Can you work these out from the model? Positions are in its coordinate system, mm. A direction names the side the tool comes from. Round coordinates to 2 decimals unless told otherwise and drop trailing zeros. Loops run counter-clockwise (first coordinate to the right, second up) from the corner with the lowest first, then second, coordinate; pieces in that order, holes last.
(1) Thinking about a two-plate mould opening in Y: for faces 5 (the face through (-2, 50.8, 135)), 6 (the face through (-2, 49, 19.05)), 7 (the face through (1.6, 47.6, 69)), which applies, released by +Y, released by -Y, zero draft, split by the parting line, or undercut?
(2) If I drill on line 1 along Z through (x, y) = (25, 34) (3 decimals); line 2 along Z through (x, y) = (38.5, 17) (3 decimals); line 3 along X through (y, z) = (3, 25) (3 decimals), over which ranges is the centre line in solid material (lowest first)?
(3) I want a section at A-A on z = 100. Write out the boundary of the cut face in (x, y) (3 decimals).
(4) Will these pins go through, and if not, where does the flat tip stop? pin 1 Ø1.9 at (x, z) = (25, 135.5) entering from +Y; pin 2 Ø4 at (x, z) = (26.5, 124) entering from +Y (3 decimals); pin 3 Ø1.6 at (y, z) = (49.5, 12.5) entering from -X.
(5) Which directions (+Z, -Z, +X, -X, +Y, -Y) give clear straight access to the entire face, cutting with the end or side of a thin tool? Please do faces 1 (the face through (-6, 25, 134.938)), 2 (the face through (22, 20.671, 135)), 3 (the face through (-2, 47.625, 97)), 4 (the face through (-6, 44.45, 137)).
(6) I want a section at C-C on x = 25.4. Write out the boundary of the cut face in (y, z) (1 decimal).
(7) I want a section at D-D on x = 42. Write out the boundary of the cut face in (y, z) (3 decimals), plus the area to 3 significant figures.
(8) I want a section at B-B on y = 28. Write out the boundary of the cut face in (x, z) (1 decimal).
from build123d import *

# Parameters (mm, degrees)
BOSS_EXTRUDE1_DEPTH = 139.7
SHELL1_T            = -3.175
BOSS_EXTRUDE2_START = -9.525
BOSS_EXTRUDE2_DEPTH = 9.525
BOSS_EXTRUDE3_DEPTH = 9.525
SKETCH5_W           = 139.7
SKETCH5_H           = 50.8
SKETCH5_W_2         = 120.65
SKETCH5_H_2         = 44.45
BOSS_EXTRUDE4_DEPTH = 3.175
SKETCH6_W           = 3.175
SKETCH6_H           = 38.1
BOSS_EXTRUDE5_DEPTH = 5.08
CUT_EXTRUDE1_REACH  = 159.09
SKETCH7_W           = 3.175
SKETCH7_H           = 9.525
SKETCH9_W           = 47.625
SKETCH9_H           = 120.65
CUT_EXTRUDE2_DEPTH  = 157.092506627
SKETCH8_R           = 0.75
BOSS_EXTRUDE6_DEPTH = 9
SKETCH10_W          = 25.4
SKETCH10_H          = 9.525
CUT_EXTRUDE3_DEPTH  = 149.683592319
SKETCH11_R          = 1.905
CUT_EXTRUDE4_DEPTH  = 25.4


with BuildPart() as part:
    # Sketch1 → Boss-Extrude1 (new body)
    with BuildSketch(Plane.XY):
        with BuildLine():
            Line((0, 0), (0, 50.8))
            ThreePointArc((0, 50.8), (35.921024484, 35.921024484), (50.8, 0))
            Line((50.8, 0), (0, 0))
        make_face()
    extrude(amount=BOSS_EXTRUDE1_DEPTH)

    # Shell1
    shell1_openings = [part.faces().sort_by_distance(p)[0] for p in [
        (0, 25.4, 69.85),
    ]]
    offset(amount=SHELL1_T, openings=shell1_openings, kind=Kind.INTERSECTION)

    # Sketch3 → Boss-Extrude2 (add)
    with BuildSketch(Plane.XY.offset(139.7).offset(BOSS_EXTRUDE2_START)):
        with BuildLine():
            Line((0, 50.8), (0, 0))
            Line((0, 0), (50.8, 0))
            ThreePointArc((50.8, 0), (35.921024484, 35.921024484), (0, 50.8))
        make_face()
    extrude(amount=BOSS_EXTRUDE2_DEPTH)

    # Sketch4 → Boss-Extrude3 (add)
    with BuildSketch(Plane(origin=(0, 0, 0), x_dir=(-1, 0, 0), z_dir=(0, 0, -1))):
        with BuildLine():
            Line((-50.8, 0), (0, 0))
            Line((0, 0), (0, 50.8))
            ThreePointArc((0, 50.8), (-35.921024484, 35.921024484), (-50.8, 0))
        make_face()
    extrude(amount=-BOSS_EXTRUDE3_DEPTH)

    # Sketch5 → Boss-Extrude4 (add)
    with BuildSketch(Plane.ZY):
        with Locations((69.85, 25.4)):
            Rectangle(SKETCH5_W, SKETCH5_H)
        with Locations((69.85, 25.4)):
            Rectangle(SKETCH5_W_2, SKETCH5_H_2, mode=Mode.SUBTRACT)
    extrude(amount=BOSS_EXTRUDE4_DEPTH)

    # Sketch6 → Boss-Extrude5 (add)
    with BuildSketch(Plane.ZY.offset(3.175)):
        with Locations((3.175, 25.4)):
            Rectangle(SKETCH6_W, SKETCH6_H)
        with Locations((136.525, 25.4)):
            Rectangle(SKETCH6_W, SKETCH6_H)
    extrude(amount=BOSS_EXTRUDE5_DEPTH)

    # Cut-Extrude1: up to this face of the body (flat: up to its plane)
    cut_extrude1_end = Plane(part.part.faces().sort_by_distance((-1.5875, 47.625, 69.85))[0])
    # Sketch7 → Cut-Extrude1 (cut, up to the picked face)
    with BuildSketch(Plane(origin=(0, 50.8, 0), x_dir=(1, 0, 0), z_dir=(0, 1, 0)), mode=Mode.PRIVATE) as cut_extrude1_sk1:
        with Locations((-1.5875, -14.2875)):
            Rectangle(SKETCH7_W, SKETCH7_H)
    cut_extrude1_tool1 = split(extrude(cut_extrude1_sk1.sketch, amount=-CUT_EXTRUDE1_REACH, mode=Mode.PRIVATE), bisect_by=cut_extrude1_end, keep=Keep.BOTH, mode=Mode.PRIVATE)
    # Sketch7 → Cut-Extrude1 (cut, up to the picked face)
    with BuildSketch(Plane(origin=(0, 50.8, 0), x_dir=(1, 0, 0), z_dir=(0, 1, 0)), mode=Mode.PRIVATE) as cut_extrude1_sk2:
        with Locations((-1.5875, -69.6595)):
            Rectangle(SKETCH7_W, SKETCH7_H)
    cut_extrude1_tool2 = split(extrude(cut_extrude1_sk2.sketch, amount=-CUT_EXTRUDE1_REACH, mode=Mode.PRIVATE), bisect_by=cut_extrude1_end, keep=Keep.BOTH, mode=Mode.PRIVATE)
    # Sketch7 → Cut-Extrude1 (cut, up to the picked face)
    with BuildSketch(Plane(origin=(0, 50.8, 0), x_dir=(1, 0, 0), z_dir=(0, 1, 0)), mode=Mode.PRIVATE) as cut_extrude1_sk3:
        with Locations((-1.5875, -125.0315)):
            Rectangle(SKETCH7_W, SKETCH7_H)
    cut_extrude1_tool3 = split(extrude(cut_extrude1_sk3.sketch, amount=-CUT_EXTRUDE1_REACH, mode=Mode.PRIVATE), bisect_by=cut_extrude1_end, keep=Keep.BOTH, mode=Mode.PRIVATE)
    add(cut_extrude1_tool1.solids().sort_by(Axis((-1.5875, 50.8, 14.2875), (0, -1, 0)))[0], mode=Mode.SUBTRACT)
    add(cut_extrude1_tool2.solids().sort_by(Axis((-1.5875, 50.8, 69.6595), (0, -1, 0)))[0], mode=Mode.SUBTRACT)
    add(cut_extrude1_tool3.solids().sort_by(Axis((-1.5875, 50.8, 125.0315), (0, -1, 0)))[0], mode=Mode.SUBTRACT)

    # Sketch9 → Cut-Extrude2 (cut, through all)
    with BuildSketch(Plane(origin=(0, 3.175, 0), x_dir=(1, 0, 0), z_dir=(0, 1, 0))):
        with Locations((26.9875, -69.85)):
            Rectangle(SKETCH9_W, SKETCH9_H)
    extrude(amount=CUT_EXTRUDE2_DEPTH, mode=Mode.SUBTRACT)

    # Sketch8 → Boss-Extrude6 (add)
    with BuildSketch(Plane(origin=(0, 3.175, 0), x_dir=(1, 0, 0), z_dir=(0, 1, 0))):
        with Locations(Location((34.373685984, -124.592684636, 0), (0, 0, 270))):
            Circle(SKETCH8_R)
        with Locations(Location((34.373685984, -58.592684636, 0), (0, 0, 270))):
            Circle(SKETCH8_R)
        with Locations(Location((9.373685984, -58.592684636, 0), (0, 0, 270))):
            Circle(SKETCH8_R)
        with Locations(Location((9.373685984, -124.592684636, 0), (0, 0, 270))):
            Circle(SKETCH8_R)
    extrude(amount=BOSS_EXTRUDE6_DEPTH)

    # Sketch10 → Cut-Extrude3 (cut, through all)
    with BuildSketch(Plane(origin=(0, 0, 130.175), x_dir=(-1, 0, 0), z_dir=(0, 0, -1))):
        with Locations((-22.088336315, 15.908721759)):
            Rectangle(SKETCH10_W, SKETCH10_H)
    extrude(amount=-CUT_EXTRUDE3_DEPTH, mode=Mode.SUBTRACT)

    # Sketch11 → Cut-Extrude4 (cut)
    with BuildSketch(Plane(origin=(0, 50.8, 0), x_dir=(1, 0, 0), z_dir=(0, 1, 0))):
        with Locations(Location((25.4, -4.7625, 0), (0, 0, 270))):
            Circle(SKETCH11_R)
        with Locations(Location((25.4, -134.9375, 0), (0, 0, 270))):
            Circle(SKETCH11_R)
    extrude(amount=-CUT_EXTRUDE4_DEPTH, mode=Mode.SUBTRACT)


solid = part.part
Filled sheet:
1. face 5: released by +Y
1. face 6: zero draft
1. face 7: undercut
2. line 1: z = 0 to 2.9, 6.625 to 9.525, 130.175 to 133.075, 136.8 to 139.7
2. line 2: z = 0 to 9.525, 130.175 to 139.7
2. line 3: x = -3.175 to 50.711
3. outline: (-3.175, 0) - (50.8, 0) arc R50.8 ccw to (50.701, 3.175) - (-3.175, 3.175) - close; (-3.175, 47.625) - (0, 47.625) arc R47.625 cw to (3.175, 47.519) - (3.175, 50.701) arc R50.8 ccw to (0, 50.8) - (-3.175, 50.8) - close
4. pin 1: stops at y = 25.4
4. pin 2: stops at y = 3.175
4. pin 3: stops at x = 0
5. face 1: -X, +Y, -Y
5. face 2: +Z
5. face 3: -X
5. face 4: +Z, -Z, -X, +Y
6. outline: (0, 0) - (44, 0) - (44, 2.9) - (25.4, 2.9) - (25.4, 6.7) - (44, 6.7) - (44, 9.5) - (3.2, 9.5) - (3.2, 130.2) - (11.1, 130.2) - (11.1, 139.7) - (0, 139.7) - close; (20.7, 130.2) - (44, 130.2) - (44, 133) - (25.4, 133) - (25.4, 136.8) - (44, 136.8) - (44, 139.7) - (20.7, 139.7) - close
7. outline: (0, 0) - (28.577, 0) - (28.577, 9.525) - (3.175, 9.525) - (3.175, 130.175) - (28.577, 130.175) - (28.577, 139.7) - (0, 139.7) - close
7. area: 927 mm2
8. outline: (-8.3, 1.6) - (-3.2, 1.6) - (-3.2, 0) - (42.4, 0) - (42.4, 9.5) - (-3.2, 9.5) - (-3.2, 4.8) - (-8.3, 4.8) - close; (-8.3, 134.9) - (-3.2, 134.9) - (-3.2, 130.2) - (42.4, 130.2) - (42.4, 139.7) - (-3.2, 139.7) - (-3.2, 138.1) - (-8.3, 138.1) - close; hole circle Ø3.8 at (25.4, 4.8); hole circle Ø3.8 at (25.4, 134.9)
